Input: part model. Units: mm. Frame: model coordinates. Coordinates: 2 decimals unless noted, no trailing zeros. Order: outer loops, then holes, each group sorted by start corner. A loop starts at its lowest first (then second) coordinate and runs counter-clockwise, first axis right, second up. Notation, with made-up numbers: (60, -5) - (106, -5) arc R25 ccw to (106, 14) - close; hole circle Ø9 at (-22, 35). An arc over 180 degrees is marked (long way). Answer as CSV lines item,"result". Start each with the question number.
Item 1: Section D-D (z = 322.5). Output: boundary loops of the cut face in (x, y), and give its area (3 significant figures).
Item 2: First-contact query: pin 1 (12 mm diameter, centred on x = -29, z = 1, fed in from +Y); pin 2 (6 mm diameter, centred on x = -41, y = -159.5, fed in from -Z); pin 3 (3 mm diameter, centred on x = 22.5, y = -62.5, fed in from +Z); pin 4 (1 mm diameter, centred on y = -166, z = 23.5, fed in from -X). Flat tips, straight axial feed; report the tip coordinate or a pass-through.
Item 3: Section B-B (x = 0). Output: boundary loops of the cut face in (y, z).
Item 4: Draft query along Z for faces 1 (the cylindrical face through (-25.37, -125.22, -19.46)), 2 (the flat face through (64.076, -229, 147)), 3 (the cylindrical face through (1.409, -228.956, 363.133)), 4 (the cylindrical face through (29.567, -125.222, -56.846)). Return one class per face: +Z half, -Z half, draft (parallel to the pull), parting line (faces both ways), or undercut.
Item 5: Section C-C (y = -41). Output: boundary loops of the cut face in (x, z), and give its area (3 significant figures).
Item 6: Material intervals for line 1 along Z through (x, y) = (0, -224); line 2 along Y through (x, z) = (50, 320.5); line 3 along Z through (x, y) = (-12, -18), sorted ascending.
Item 7: Section A-A (z = 85.5). Output: boundary loops of the cut face in (x, y).
from build123d import *

# Parameters (mm, degrees)
F0_R     = 64.0760449632
F0_R_2   = 31.9745078145
F1_DEPTH = 254
F2_R     = 31.9745078145
F3_DEPTH = 50.8
F4_R     = 31.9745078145
F5_DEPTH = 50.8


with BuildPart() as f1:
    # F0 (on Front) → F1 (new body)
    with BuildSketch(Plane.XZ):
        Circle(F0_R)
        Circle(F0_R_2, mode=Mode.SUBTRACT)
    extrude(amount=F1_DEPTH)

    # F2 (on face) → F3 (join)
    with BuildSketch(Plane(origin=(0, 0, 0), x_dir=(-1, 0, 0), z_dir=(0, 1, 0))):
        with BuildLine():
            ThreePointArc((-64.0760449632, 0), (0, -64.0760449632), (64.0760449632, 0))
            ThreePointArc((64.0760449632, 0), (0, 64.0760449632), (-64.0760449632, 0))
        make_face()
        Circle(F2_R, mode=Mode.SUBTRACT)
        with BuildLine():
            ThreePointArc((-64.0760449632, 0), (0, 64.0760449632), (64.0760449632, 0))
            Line((64.0760449632, 0), (64.0760449632, 299.0727424622))
            ThreePointArc((64.0760449632, 299.0727424622), (0, 363.1487874254), (-64.0760449632, 299.0727424622))
            Line((-64.0760449632, 299.0727424622), (-64.0760449632, 0))
        make_face()
        with Locations((0, 299.0727424622)):
            Circle(F2_R, mode=Mode.SUBTRACT)
    extrude(amount=-F3_DEPTH)

    # F4 (on face) → F5 (join)
    with BuildSketch(Plane.XZ.offset(254)):
        with BuildLine():
            Line((64.0760449632, 0), (64.0760449632, 299.0727424622))
            ThreePointArc((64.0760449632, 299.0727424622), (0, 363.1487874254), (-64.0760449632, 299.0727424622))
            Line((-64.0760449632, 299.0727424622), (-64.0760449632, 0))
            ThreePointArc((-64.0760449632, 0), (0, 64.0760449632), (64.0760449632, 0))
        make_face()
        with Locations((0, 299.0727424622)):
            Circle(F4_R, mode=Mode.SUBTRACT)
    extrude(amount=-F5_DEPTH)


solid = f1.part
Determined:
1,outline,"(-59.64, -254) - (-21.76, -254) - (-21.76, -203.2) - (-59.64, -203.2) - close; (-59.64, -50.8) - (-21.76, -50.8) - (-21.76, 0) - (-59.64, 0) - close; (21.76, -254) - (59.64, -254) - (59.64, -203.2) - (21.76, -203.2) - close; (21.76, -50.8) - (59.64, -50.8) - (59.64, 0) - (21.76, 0) - close"
1,area,"7,700 mm^2"
2,pin 1,"stops at y = 0"
2,pin 2,"stops at z = -51.59"
2,pin 3,"stops at z = 60.54"
2,pin 4,"stops at x = -59.81"
3,outline,"(-254, -64.08) - (0, -64.08) - (0, -31.97) - (-254, -31.97) - close; (-254, 31.97) - (0, 31.97) - (0, 267.1) - (-50.8, 267.1) - (-50.8, 64.08) - (-203.2, 64.08) - (-203.2, 267.1) - (-254, 267.1) - close; (-254, 331.05) - (-203.2, 331.05) - (-203.2, 363.15) - (-254, 363.15) - close; (-50.8, 331.05) - (0, 331.05) - (0, 363.15) - (-50.8, 363.15) - close"
4,face 1,"undercut"
4,face 2,"draft"
4,face 3,"+Z half"
4,face 4,"parting line"
5,outline,"(-64.08, 0) arc R64.08 ccw to (64.08, 0) - (64.08, 299.07) arc R64.08 ccw to (-64.08, 299.07) - close; hole circle Ø63.95 at (0, 0); hole circle Ø63.95 at (0, 299.07)"
5,area,"44,800 mm^2"
6,line 1,"z = -64.08 to -31.97, 31.97 to 267.1, 331.05 to 363.15"
6,line 2,"y = -254 to -203.2, -50.8 to 0"
6,line 3,"z = -62.94 to -29.64, 29.64 to 269.44, 328.71 to 362.02"
7,outline,"(-64.08, -254) - (64.08, -254) - (64.08, -203.2) - (-64.08, -203.2) - close; (-64.08, -50.8) - (64.08, -50.8) - (64.08, 0) - (-64.08, 0) - close"
